from build123d import *

# Parameters (mm, degrees)
BOSS_EXTRUDE1_DEPTH      = 55.499
SKETCH2_R                = 12.6492
CUT_EXTRUDE1_DEPTH       = 21.082
CUT_EXTRUDE2_START       = -47.498
CUT_EXTRUDE2_DEPTH       = 47.498
CUT_EXTRUDE3_DEPTH       = 64.719756461
CUT_EXTRUDE4_DEPTH       = 69.159299334
CUT_EXTRUDE5_DEPTH       = 69.159299334
FILLET1_R                = 4.9911
FILLET2_R                = 4.9911
SKETCH7_R                = 1.27
CUT_EXTRUDE6_DEPTH       = 4.826
CUT_EXTRUDE7_START       = -4.826
SKETCH8_R                = 1.27
CUT_EXTRUDE7_DEPTH       = 4.826
SKETCH9_R                = 1.27
CUT_EXTRUDE8_DEPTH       = 4.318
CUT_EXTRUDE9_START       = -4.318
SKETCH10_R               = 1.27
CUT_EXTRUDE9_DEPTH       = 4.318
SKETCH11_W               = 1.6764
SKETCH11_H               = 7.62
CUT_EXTRUDE10_DEPTH      = 69.159299334
BOSS_EXTRUDE2_DEPTH      = 8.0772
SKETCH13_W               = 1.27
SKETCH13_H               = 8.69888745
CUT_EXTRUDE11_DEPTH      = 8.0772
FILLET3_R                = 1.5875
SKETCH14_R               = 1.27
CUT_EXTRUDE12_DEPTH      = 67.881616192
SKETCH15_R               = 2.032
CUT_EXTRUDE13_DEPTH      = 0.889
CUT_EXTRUDE14_START      = -0.889
SKETCH16_R               = 2.032
CUT_EXTRUDE14_DEPTH      = 0.889
SCALE1_SCALE             = 0.6
CUT_EXTRUDE15_DEPTH      = 51.873928307
CUT_EXTRUDE15_DEPTH_BACK = 51.873928307
SKETCH17_W               = 22.594181605
SKETCH17_H               = 22.052877317
SKETCH18_W               = 16.764
SKETCH18_H               = 50
BOSS_EXTRUDE3_DEPTH      = 2.5
FILLET4_R                = 8
M3_CLEARANCE_HOLE1_D     = 3.4
M3_CLEARANCE_HOLE1_DEPTH = 2.5


with BuildPart() as part:
    # Sketch1 → Boss-Extrude1 (new body)
    with BuildSketch(Plane.XY):
        with BuildLine():
            Line((-13.97, 0), (13.97, 0))
            Line((13.97, 0), (13.97, 17.415057792))
            ThreePointArc((13.97, 17.415057792), (13.699370909, 17.834675567), (13.502160632, 18.293399109))
            ThreePointArc((13.502160632, 18.293399109), (0, 28.0162), (-13.502160632, 18.293399109))
            ThreePointArc((-13.502160632, 18.293399109), (-13.699370909, 17.834675567), (-13.97, 17.415057792))
            Line((-13.97, 17.415057792), (-13.97, 0))
        make_face()
    extrude(amount=-BOSS_EXTRUDE1_DEPTH)

    # Sketch2 → Cut-Extrude1 (cut)
    with BuildSketch(Plane.XY):
        with Locations((0, 13.7795)):
            Circle(SKETCH2_R)
    extrude(amount=-CUT_EXTRUDE1_DEPTH, mode=Mode.SUBTRACT)

    # Sketch3 → Cut-Extrude2 (cut)
    with BuildSketch(Plane(origin=(0, 0, -55.499), x_dir=(-1, 0, 0), z_dir=(0, 0, -1)).offset(CUT_EXTRUDE2_START)):
        with BuildLine():
            Line((-13.97, 0), (-13.97, 11.036741008))
            ThreePointArc((-13.97, 11.036741008), (-10.365518606, 4.020419566), (-3.578967259, 0))
            Line((-3.578967259, 0), (-13.97, 0))
        make_face()
        with BuildLine():
            Line((13.97, 0), (3.578967259, 0))
            ThreePointArc((3.578967259, 0), (10.365518606, 4.020419566), (13.97, 11.036741008))
            Line((13.97, 11.036741008), (13.97, 0))
        make_face()
    extrude(amount=CUT_EXTRUDE2_DEPTH, mode=Mode.SUBTRACT)

    # Sketch4 → Cut-Extrude3 (cut, through all)
    with BuildSketch(Plane(origin=(0, 0, 0), x_dir=(1, 0, 0), z_dir=(0, 1, 0))):
        with BuildLine():
            Line((-10.033, 46.5201), (-10.033, 26.4795))
            ThreePointArc((-10.033, 26.4795), (-8.861280678, 23.650719322), (-6.0325, 22.479))
            Line((-6.0325, 22.479), (6.0325, 22.479))
            ThreePointArc((6.0325, 22.479), (8.861280678, 23.650719322), (10.033, 26.4795))
            Line((10.033, 26.4795), (10.033, 46.5201))
            ThreePointArc((10.033, 46.5201), (8.861280678, 49.348880678), (6.0325, 50.5206))
            Line((6.0325, 50.5206), (-6.0325, 50.5206))
            ThreePointArc((-6.0325, 50.5206), (-8.861280678, 49.348880678), (-10.033, 46.5201))
        make_face()
    extrude(amount=CUT_EXTRUDE3_DEPTH, mode=Mode.SUBTRACT)

    # Sketch5 → Cut-Extrude4 (cut, through all)
    with BuildSketch(Plane(origin=(13.97, 0, 0), x_dir=(0, 0, -1), z_dir=(1, 0, 0))):
        with BuildLine():
            Line((22.479, 30.552887158), (22.479, 23.126200001))
            ThreePointArc((22.479, 23.126200001), (23.650572876, 20.297772876), (26.479000001, 19.1262))
            Line((26.479000001, 19.1262), (58.380075255, 19.1262))
            Line((58.380075255, 19.1262), (58.380075255, 30.552887158))
            Line((58.380075255, 30.552887158), (22.479, 30.552887158))
        make_face()
    extrude(amount=-CUT_EXTRUDE4_DEPTH, mode=Mode.SUBTRACT)

    # Sketch6 → Cut-Extrude5 (cut, through all)
    with BuildSketch(Plane(origin=(13.97, 0, 0), x_dir=(0, 0, -1), z_dir=(1, 0, 0))):
        with BuildLine():
            Line((26.479000001, 5.7404), (41.275, 5.7404))
            Line((41.275, 5.7404), (56.850797395, 10.801283358))
            Line((56.850797395, 10.801283358), (56.850797395, -1.681383137))
            Line((56.850797395, -1.681383137), (22.479, -1.681383137))
            Line((22.479, -1.681383137), (22.479, 1.740399999))
            ThreePointArc((22.479, 1.740399999), (23.650572876, 4.568827124), (26.479000001, 5.7404))
        make_face()
    extrude(amount=-CUT_EXTRUDE5_DEPTH, mode=Mode.SUBTRACT)

    # Fillet1
    fillet1_edges = [part.edges().sort_by_distance(p)[0] for p in [
        (0, 19.1262, -55.499),
    ]]
    fillet(fillet1_edges, radius=FILLET1_R)

    # Fillet2
    fillet2_edges = [part.edges().sort_by_distance(p)[0] for p in [
        (0, 10.362057759, -55.499),
    ]]
    fillet(fillet2_edges, radius=FILLET2_R)

    # Sketch7 → Cut-Extrude6 (cut)
    with BuildSketch(Plane(origin=(13.97, 0, 0), x_dir=(0, 0, -1), z_dir=(1, 0, 0))):
        with Locations(Location((50.5079, 14.061702085, 0), (0, 0, 90))):
            Circle(SKETCH7_R)
    extrude(amount=-CUT_EXTRUDE6_DEPTH, mode=Mode.SUBTRACT)

    # Sketch8 → Cut-Extrude7 (cut)
    with BuildSketch(Plane.ZY.offset(13.97).offset(CUT_EXTRUDE7_START)):
        with Locations(Location((-50.5079, 14.061702085, 0), (0, 0, 90))):
            Circle(SKETCH8_R)
    extrude(amount=CUT_EXTRUDE7_DEPTH, mode=Mode.SUBTRACT)

    # Sketch9 → Cut-Extrude8 (cut)
    with BuildSketch(Plane(origin=(13.97, 0, 0), x_dir=(0, 0, -1), z_dir=(1, 0, 0))):
        with Locations(Location((4.0005, 4.1148, 0), (0, 0, 90))):
            Circle(SKETCH9_R)
    extrude(amount=-CUT_EXTRUDE8_DEPTH, mode=Mode.SUBTRACT)

    # Sketch10 → Cut-Extrude9 (cut)
    with BuildSketch(Plane.ZY.offset(13.97).offset(CUT_EXTRUDE9_START)):
        with Locations(Location((-4.0005, 4.1148, 0), (0, 0, 90))):
            Circle(SKETCH10_R)
    extrude(amount=CUT_EXTRUDE9_DEPTH, mode=Mode.SUBTRACT)

    # Sketch11 → Cut-Extrude10 (cut, through all)
    with BuildSketch(Plane.ZY.offset(13.97)):
        with Locations((-8.9154, 24.2062)):
            Rectangle(SKETCH11_W, SKETCH11_H)
    extrude(amount=-CUT_EXTRUDE10_DEPTH, mode=Mode.SUBTRACT)

    # Sketch12 → Boss-Extrude2 (add)
    with BuildSketch(Plane.XY):
        with BuildLine():
            Line((-3.6195, 32.9184), (3.6195, 32.9184))
            Line((3.6195, 32.9184), (3.6195, 27.548408695))
            ThreePointArc((3.6195, 27.548408695), (0, 28.0162), (-3.6195, 27.548408695))
            Line((-3.6195, 27.548408695), (-3.6195, 32.9184))
        make_face()
    extrude(amount=-BOSS_EXTRUDE2_DEPTH)

    # Sketch13 → Cut-Extrude11 (cut)
    with BuildSketch(Plane.XY):
        with Locations((1.4351, 29.199787514)):
            Rectangle(SKETCH13_W, SKETCH13_H)
    extrude(amount=-CUT_EXTRUDE11_DEPTH, mode=Mode.SUBTRACT)

    # Fillet3
    fillet3_edges = [part.edges().sort_by_distance(p)[0] for p in [
        (3.6195, 27.548408695, -4.0386),
        (-3.6195, 27.548408695, -4.0386),
    ]]
    fillet(fillet3_edges, radius=FILLET3_R)

    # Sketch14 → Cut-Extrude12 (cut, through all)
    with BuildSketch(Plane(origin=(3.6195, 0, 0), x_dir=(0, 0, -1), z_dir=(1, 0, 0))):
        with Locations(Location((4.0386, 30.820436744, 0), (0, 0, 90))):
            Circle(SKETCH14_R)
    extrude(amount=-CUT_EXTRUDE12_DEPTH, mode=Mode.SUBTRACT)

    # Sketch15 → Cut-Extrude13 (cut)
    with BuildSketch(Plane(origin=(13.97, 0, 0), x_dir=(0, 0, -1), z_dir=(1, 0, 0))):
        with Locations(Location((4.0005, 4.1148, 0), (0, 0, 90))):
            Circle(SKETCH15_R)
        with Locations(Location((50.5079, 14.061702085, 0), (0, 0, 90))):
            Circle(SKETCH15_R)
    extrude(amount=-CUT_EXTRUDE13_DEPTH, mode=Mode.SUBTRACT)

    # Sketch16 → Cut-Extrude14 (cut)
    with BuildSketch(Plane.ZY.offset(13.97).offset(CUT_EXTRUDE14_START)):
        with Locations(Location((-50.5079, 14.061702085, 0), (0, 0, 90))):
            Circle(SKETCH16_R)
        with Locations(Location((-4.0005, 4.1148, 0), (0, 0, 90))):
            Circle(SKETCH16_R)
    extrude(amount=CUT_EXTRUDE14_DEPTH, mode=Mode.SUBTRACT)


with BuildPart() as part_1:
    # Scale1: scaled about (-0.010832485, 13.272964488, -25.431393294)
    add(part.part.scale(SCALE1_SCALE).moved(Location((-0.004332994, 5.309185795, -10.172557318))))

    # Sketch17 → Cut-Extrude15 (cut, two sides: drawn at the far end of the back side and taken through both)
    with BuildSketch(Plane(origin=(0, 0, 0), x_dir=(1, 0, 0), z_dir=(0, 1, 0)).offset(-CUT_EXTRUDE15_DEPTH_BACK)):
        with Locations((1.099382363, 34.686357372)):
            Rectangle(SKETCH17_W, SKETCH17_H)
    extrude(amount=CUT_EXTRUDE15_DEPTH + CUT_EXTRUDE15_DEPTH_BACK, mode=Mode.SUBTRACT)

    # Sketch18 → Boss-Extrude3 (add)
    with BuildSketch(Plane(origin=(0, 0, -23.659918713), x_dir=(-1, 0, 0), z_dir=(0, 0, -1))):
        with Locations((0.004315992, 13.576876814)):
            Rectangle(SKETCH18_W, SKETCH18_H)
    extrude(amount=BOSS_EXTRUDE3_DEPTH)

    # Fillet4
    fillet4_edges = [part_1.edges().sort_by_distance(p)[0] for p in [
        (8.377684008, 38.576876814, -24.909918713),
        (8.377684008, -11.423123186, -24.909918713),
        (-8.386315992, -11.423123186, -24.909918713),
        (-8.386315992, 38.576876814, -24.909918713),
    ]]
    fillet(fillet4_edges, radius=FILLET4_R)

    # M3 Clearance Hole1
    with Locations(Plane.XY.offset(-23.659918713)):
        with Locations((-0.004315992, 26.576876814), (-0.004315992, -7.423123186), (-0.004315992, 0.576876814), (-0.004315992, 34.576876814)):
            Hole(M3_CLEARANCE_HOLE1_D / 2, depth=M3_CLEARANCE_HOLE1_DEPTH)


solid = part_1.part
Geometry: final body of the model. Coordinates: model frame, mm. A direction names the side the tool comes from. Give positions to 0.01 mm unless a question says otherwise; leave off trailing zeros. Loops run counter-clockwise (first coordinate to the right, second up) from the corner with the lowest first, then second, coordinate; pieces in that order, holes last. Notation, with made-up numbers: M 44.5,13.25 L 63.5,13.25 A26 ccw 63.5,29.25 Z; hole C 65.25,88.25 d9. An arc over 180 degrees is marked long. Put each result on its own line as item: value.
1) Material intervals for L1, parallel to X at y = 13.5, z = -11.25; L2, parallel to Y at x = -1, z = -25.25; L3, parallel to Z at x = 6, y = 15, sorted ascending. Write a range as from..to.
Computed values:
L1: x = -8.39..-7.59, 7.58..8.38
L2: y = -11.4..-8.8, -6.05..-0.8, 1.95..25.2, 27.95..33.2, 35.95..38.55
L3: z = -26.16..-22.82
2) Mould query, pull axis Y, two halves, no side actions, for faces 1 (the cylindrical face through (0.22, 36.26, -24.93)), 2 (the cylindrical face through (6.1, 36.17, -24.93)), 3 (the cylindrical face through (6.096, -9.017, -24.927)). Classes: released by +Y, released by -Y, zero draft, split by the parting line, or undercut.
Computed values:
face 1: undercut
face 2: released by +Y
face 3: released by -Y
3) First-contact query: P1, Ø1.2, axis at y = 7.5, z = -12.5, coming from the -X side; P2, Ø4.5, axis at y = 22.5, z = -12.5, coming from the +X side; P3, Ø2, axis at y = 23.5, z = -13, coming from the -X side; P4, Ø6, axis at y = 0.5, z = -18.5, coming from the +X side. Flat tips, straight axial feed; report the tip coordinate or a pass-through.
Computed values:
P1: stops at x = -7.85
P2: stops at x = 5.33
P3: stops at x = -2.18
P4: passes through
4) Cut plane C-C, the plane y = 24. Return the cut outline in (x, z).
Computed values:
outline: M -8.39,-26.16 L 8.38,-26.16 L 8.38,-23.66 L -8.39,-23.66 Z; M -2.18,-15.02 L 0.48,-15.02 L 0.48,-13.33 L -2.18,-13.33 Z; M -2.18,-11.86 L 0.48,-11.86 L 0.48,-10.17 L -2.18,-10.17 Z; M 1.24,-15.02 L 2.17,-15.02 L 2.17,-13.33 L 1.24,-13.33 Z; M 1.24,-11.86 L 2.17,-11.86 L 2.17,-10.17 L 1.24,-10.17 Z
5) Cut plane B-B, the plane z = -17. Return the cut outline in (x, y).
Computed values:
outline: M -8.39,11.93 A8.54 ccw -2.15,5.31 L 2.14,5.31 A8.54 ccw 8.38,11.93 L 8.38,15.76 A1.8 cw 8.1,16.29 A8.54 ccw -8.11,16.29 A1.8 cw -8.39,15.76 Z; hole C 0,13.58 d15.18
6) Cut plane D-D, the plane z = -24.75. Return the cut outline in (x, y).
Computed values:
outline: M -8.39,-3.42 A8 ccw -0.39,-11.42 L 0.38,-11.42 A8 ccw 8.38,-3.42 L 8.38,30.58 A8 ccw 0.38,38.58 L -0.39,38.58 A8 ccw -8.39,30.58 Z; hole C 0,-7.42 d3.4; hole C 0,0.58 d3.4; hole C 0,26.58 d3.4; hole C 0,34.58 d3.4
7) Cut plane A-A, the plane x = 3.25. Return the cut outline in (y, z), plus the area to 3 significant figures.
Computed values:
outline: M -10.89,-26.16 L 38.04,-26.16 L 38.04,-23.66 L 21.47,-23.66 L 21.47,-16.02 L 20.43,-16.02 L 20.43,-22.82 L 6.72,-22.82 L 6.72,-10.17 L 5.31,-10.17 L 5.31,-14.97 L 5.68,-14.97 L 5.68,-23.66 L -10.89,-23.66 Z; M 20.43,-15.02 L 21.47,-15.02 L 21.47,-10.17 L 20.43,-10.17 Z
area: 163 mm^2
8) Reachability of faces 4 (the flat face through (-7, 7, -14.973)), 5 (the flat face through (2.167, 23, -12)), 6 (the flat face through (2, 25.06, -13)), 7 (the flat face through (5.787, 8, -13)), 8 (the flat face through (3.9, 21, -15.019)) from +Z, -Z, +X, -X, +Y, -Y: full face, straight path, thin tool, end or side. Return the list, or none.
Computed values:
face 4: -X, -Y
face 5: +Z, +X, +Y
face 6: +Z, +X, -X, +Y
face 7: +X
face 8: +X, -X, +Y
